```python
from build123d import *

# Parameters (mm, degrees)
BOSS_EXTRU_1_DEPTH                       = 28.5
ESQUISSE5_W                              = 45
ESQUISSE5_H                              = 12.6
BOSS_EXTRU_2_DEPTH                       = 9
ESQUISSE3_R                              = 24.1
ENL_V_MAT_EXTRU_3_DEPTH                  = 8
ENL_V_START                              = -12.6
ENL_V_MAT_EXTRU_5_DEPTH                  = 12.6
ENL_V_START_2                            = -1
ESQUISSE4_R                              = 24.1
ESQUISSE4_R_2                            = 8.05
ENL_V_MAT_EXTRU_4_DEPTH                  = 1
ENL_V_MAT_EXTRU_7_DEPTH                  = 161.796665884
ENL_V_MAT_EXTRU_7_DEPTH_BACK             = 161.796665884
ENL_V_START_3                            = -4
ESQUISSE8_R                              = 7.5
ENL_V_MAT_EXTRU_8_DEPTH                  = 26
ENL_V_START_4                            = 8
ESQUISSE9_R                              = 15
ENL_V_MAT_EXTRU_9_DEPTH                  = 10
ESQUISSE10_R                             = 15
ESQUISSE10_R_2                           = 8.05
ENL_V_MAT_EXTRU_10_DEPTH                 = 1
CONG_1_R                                 = 2
ESQUISSE11_W                             = 12
ESQUISSE11_H                             = 8
ENL_V_MAT_EXTRU_11_DEPTH                 = 23.5
CONG_2_R                                 = 1
FRAISAGE_POUR_VIS_T_TE_FRAIS_E_6_2_COUNT = 2
FRAISAGE_POUR_VIS_T_TE_FRAIS_E_6_2_PITCH = 48
ESQUISSE16_R                             = 1.35
ENL_V_MAT_EXTRU_12_DEPTH                 = 7
BOSS_EXTRU_4_START                       = 1.75
BOSS_EXTRU_4_DEPTH                       = 1.75
BOSS_EXTRU_5_DEPTH                       = 1.75
CHANFREIN2_ANGLE                         = 177.039506
CHANFREIN1_SIZE                          = 1.5


with BuildPart() as part:
    # Esquisse1 → Boss.-Extru.1 (new body)
    with BuildSketch(Plane(origin=(0, -156.353982231, 0), x_dir=(1, 0, 0), z_dir=(0, 1, 0))):
        with BuildLine():
            Line((16.5, -20), (16.5, 20))
            ThreePointArc((16.5, 20), (15.792893219, 20.292893219), (15.5, 21))
            Line((15.5, 21), (15.5, 24))
            ThreePointArc((15.5, 24), (11.5, 28), (7.5, 24))
            Line((7.5, 24), (7.5, 18.75))
            Line((7.5, 18.75), (7.5, 17))
            ThreePointArc((7.5, 17), (7.207106781, 16.292893219), (6.5, 16))
            Line((6.5, 16), (-12, 16))
            ThreePointArc((-12, 16), (-12.707106781, 16.292893219), (-13, 17))
            Line((-13, 17), (-13, 24))
            ThreePointArc((-13, 24), (-17, 28), (-21, 24))
            Line((-21, 24), (-21, 21))
            ThreePointArc((-21, 21), (-21.292893219, 20.292893219), (-22, 20))
            Line((-22, 20), (-25, 20))
            Line((-25, 20), (-25, -20))
            Line((-25, -20), (-22, -20))
            ThreePointArc((-22, -20), (-21.292893219, -20.292893219), (-21, -21))
            Line((-21, -21), (-21, -24))
            ThreePointArc((-21, -24), (-17, -28), (-13, -24))
            Line((-13, -24), (-13, -13))
            ThreePointArc((-13, -13), (-12.707106781, -12.292893219), (-12, -12))
            Line((-12, -12), (6.5, -12))
            ThreePointArc((6.5, -12), (7.207106781, -12.292893219), (7.5, -13))
            Line((7.5, -13), (7.5, -24))
            ThreePointArc((7.5, -24), (11.5, -28), (15.5, -24))
            Line((15.5, -24), (15.5, -21))
            ThreePointArc((15.5, -21), (15.792893219, -20.292893219), (16.5, -20))
        make_face()
    extrude(amount=BOSS_EXTRU_1_DEPTH)

    # Esquisse5 → Boss.-Extru.2 (add)
    with BuildSketch(Plane(origin=(0, -127.853982231, 0), x_dir=(1, 0, 0), z_dir=(0, 1, 0))):
        with Locations((-2.5, 7.3)):
            Rectangle(ESQUISSE5_W, ESQUISSE5_H)
    extrude(amount=BOSS_EXTRU_2_DEPTH)

    # Esquisse3 → Enlèv. mat.-Extru.3 (cut)
    with BuildSketch(Plane(origin=(0, -128.853982231, -11), x_dir=(1, 0, 0), z_dir=(0, 0, 1))):
        with Locations((0, -15.5)):
            Circle(ESQUISSE3_R)
    extrude(amount=ENL_V_MAT_EXTRU_3_DEPTH, mode=Mode.SUBTRACT)

    # Esquisse6 → Enlèv. mat.-Extru.5 (cut)
    with BuildSketch(Plane.XY.offset(-1).offset(ENL_V_START)):
        Polygon((-25, -104.147876216), (-25, -127.853982231), (-21, -127.853982231), (-21, -123.853982231), (-6, -118.853982231), (6, -118.853982231), (20, -123.853982231), (20, -104.147876216), align=None)
    extrude(amount=ENL_V_MAT_EXTRU_5_DEPTH, mode=Mode.SUBTRACT)

    # Esquisse4 → Enlèv. mat.-Extru.4 (cut)
    with BuildSketch(Plane(origin=(0, -168.853982231, -11), x_dir=(1, 0, 0), z_dir=(0, 0, 1)).offset(ENL_V_START_2)):
        with Locations((0, 24.5)):
            Circle(ESQUISSE4_R)
        with Locations((0, 24.5)):
            Circle(ESQUISSE4_R_2, mode=Mode.SUBTRACT)
    extrude(amount=ENL_V_MAT_EXTRU_4_DEPTH, mode=Mode.SUBTRACT)

    # Esquisse7 → Enlèv. mat.-Extru.7 (cut, two sides: drawn at the far end of the back side and taken through both)
    with BuildSketch(Plane.XY.offset(-ENL_V_MAT_EXTRU_7_DEPTH_BACK)):
        with BuildLine():
            Line((-4.030508653, -148.384490884), (-12, -156.353982231))
            Line((-12, -156.353982231), (16.5, -156.353982231))
            Line((16.5, -156.353982231), (16.5, -127.853982231))
            Line((16.5, -127.853982231), (4.030508653, -140.323473578))
            ThreePointArc((4.030508653, -140.323473578), (-4.030508653, -140.323473578), (-4.030508653, -148.384490884))
        make_face()
    extrude(amount=ENL_V_MAT_EXTRU_7_DEPTH + ENL_V_MAT_EXTRU_7_DEPTH_BACK, mode=Mode.SUBTRACT)

    # Esquisse8 → Enlèv. mat.-Extru.8 (cut)
    with BuildSketch(Plane.XY.offset(-11).offset(ENL_V_START_3)):
        with Locations((0, -144.353982231)):
            Circle(ESQUISSE8_R)
    extrude(amount=ENL_V_MAT_EXTRU_8_DEPTH, mode=Mode.SUBTRACT)

    # Esquisse9 → Enlèv. mat.-Extru.9 (cut)
    with BuildSketch(Plane.XY.offset(-11).offset(ENL_V_START_4)):
        with Locations((0, -144.353982231)):
            Circle(ESQUISSE9_R)
    extrude(amount=ENL_V_MAT_EXTRU_9_DEPTH, mode=Mode.SUBTRACT)

    # Esquisse10 → Enlèv. mat.-Extru.10 (cut)
    with BuildSketch(Plane(origin=(0, 0, 7), x_dir=(-1, 0, 0), z_dir=(0, 0, -1)).offset(ENL_V_START_2)):
        with Locations((0, -144.353982231)):
            Circle(ESQUISSE10_R)
        with Locations((0, -144.353982231)):
            Circle(ESQUISSE10_R_2, mode=Mode.SUBTRACT)
    extrude(amount=ENL_V_MAT_EXTRU_10_DEPTH, mode=Mode.SUBTRACT)

    # Congé1
    # the kernel refuses this fillet: 2 mm, written as the material it adds along each edge
    with BuildSketch(Plane(origin=(0, -144.353982231, -12), x_dir=(0.7071067811865527, 0.7071067811865425, 0), z_dir=(0.7071067811865425, -0.7071067811865527, 0))) as cong_1_piece_1:
        with BuildLine():
            CenterArc((9.782050808, 2), CONG_1_R, 210, 60)
            Line((9.782050808, 0), (8.05, 0))
            Line((8.05, 0), (8.05, 1))
        make_face()
    revolve(axis=Axis((0, -144.353982231, -12), (0, 0, 1)), revolution_arc=180)
    with BuildSketch(Plane(origin=(0, -144.353982231, 8), x_dir=(0.7071067811865495, 0.7071067811865456, 0), z_dir=(0.7071067811865456, -0.7071067811865495, 0))) as cong_1_piece_2:
        with BuildLine():
            CenterArc((9.782050808, -2), CONG_1_R, 90, 60)
            Line((8.05, -1), (8.05, 0))
            Line((8.05, 0), (9.782050808, 0))
        make_face()
    revolve(axis=Axis((0, -144.353982231, 8), (0, 0, 1)), revolution_arc=180)
    # the kernel refuses this fillet: 2 mm, written as the material it takes off along each edge
    with BuildSketch(Plane(origin=(0, -144.353982231, -3), x_dir=(0.8997810894111481, 0.43634159913774845, 0), z_dir=(0.43634159913774845, -0.8997810894111481, 0))) as cong_1_2_piece_1:
        with BuildLine():
            CenterArc((15 + CONG_1_R, CONG_1_R), CONG_1_R, 180, 90)
            Line((15 + CONG_1_R, 0), (15, 0))
            Line((15, 0), (15, CONG_1_R))
        make_face()
    revolve(axis=Axis((0, -144.353982231, -3), (0, 0, 1)), revolution_arc=218.25861464, mode=Mode.SUBTRACT)

    # Esquisse11 → Enlèv. mat.-Extru.11 (cut)
    with BuildSketch(Plane(origin=(0, -127.853982231, 0), x_dir=(1, 0, 0), z_dir=(0, 1, 0))):
        with Locations((-19, 24)):
            Rectangle(ESQUISSE11_W, ESQUISSE11_H)
        with Locations((-19, -24)):
            Rectangle(ESQUISSE11_W, ESQUISSE11_H)
    extrude(amount=-ENL_V_MAT_EXTRU_11_DEPTH, mode=Mode.SUBTRACT)

    # Congé2
    cong_2_edges = [part.edges().sort_by_distance(p)[0] for p in [
        (-17.5, -151.353982231, -20),
        (-17.5, -151.353982231, 20),
    ]]
    fillet(cong_2_edges, radius=CONG_2_R)

    # Esquisse12 → Fraisage pour vis _ t_te frais_e _ 6 pan (revolve, cut)
    with BuildSketch(Plane(origin=(-17, -151.353982231, -24), x_dir=(0, 0, 1), z_dir=(1, 0, 0))):
        Polygon((0, 0), (0, 5), (1.6, 5), (1.6, 1.7), (2.9, 0.4), (2.9, 0), align=None)
    fraisage_pour_vis_t_te_frais_e_6_pan = revolve(axis=Axis((-17, -145.003982231, -24), (0, -1, 0)), mode=Mode.SUBTRACT)

    # Fraisage pour vis _ t_te frais_e _ 6 2: Fraisage pour vis _ t_te frais_e _ 6 pan ×2
    with Locations(*[(0, 0, i * FRAISAGE_POUR_VIS_T_TE_FRAIS_E_6_2_PITCH) for i in range(1, FRAISAGE_POUR_VIS_T_TE_FRAIS_E_6_2_COUNT)]):
        add(fraisage_pour_vis_t_te_frais_e_6_pan, mode=Mode.SUBTRACT)

    # Fraisage pour vis _ t_te frais_e _ 6 3: read off the stored shape, not the designer's step
    # Fraisage pour vis _ t_te frais_e _ 6 3 o → Fraisage pour vis _ t_te frais_e _ 6 3 (revolve, cut)
    with BuildSketch(Plane(origin=(11.5, 0, 24), x_dir=(1, 0, 0), z_dir=(0, 0, 1))):
        Polygon((0, -134.475881673), (1.6, -134.475881673), (1.6, -129.553982231), (2.9, -128.253982231), (2.9, -127.853982231), (0, -127.853982231), align=None)
    revolve(axis=Axis((11.5, 0, 24), (0, 1, 0)), mode=Mode.SUBTRACT)

    # Fraisage pour vis _ t_te frais_e _ 6 4 → Fraisage pour vis _ t_te frais_e _ 6 3 2 (revolve, cut)
    with BuildSketch(Plane(origin=(11.5, 0, -24), x_dir=(1, 0, 0), z_dir=(0, 0, 1))):
        Polygon((0, -134.475881673), (1.6, -134.475881673), (1.6, -129.553982231), (2.9, -128.253982231), (2.9, -127.853982231), (0, -127.853982231), align=None)
    revolve(axis=Axis((11.5, 0, -24), (0, 1, 0)), mode=Mode.SUBTRACT)

    # Esquisse16 → Enlèv. mat.-Extru.12 (cut)
    with BuildSketch(Plane(origin=(0, -127.853982231, 0), x_dir=(1, 0, 0), z_dir=(0, 1, 0))):
        with Locations(Location((-21, 16.8, 0), (0, 0, 180))):
            Circle(ESQUISSE16_R)
        with Locations(Location((11.5, 16.8, 0), (0, 0, 180))):
            Circle(ESQUISSE16_R)
        with Locations((11.5, -16.8)):
            Circle(ESQUISSE16_R)
        with Locations((-21, -16.8)):
            Circle(ESQUISSE16_R)
    extrude(amount=-ENL_V_MAT_EXTRU_12_DEPTH, mode=Mode.SUBTRACT)

    # Esquisse17 → Boss.-Extru.4 (add)
    with BuildSketch(Plane(origin=(0, 0, -16), x_dir=(-1, 0, 0), z_dir=(0, 0, -1)).offset(BOSS_EXTRU_4_START)):
        with BuildLine():
            Line((-4.030508653, -140.323473578), (-7.919595949, -136.434386282))
            ThreePointArc((-7.919595949, -136.434386282), (7.919595949, -136.434386282), (7.919595949, -152.27357818))
            Line((7.919595949, -152.27357818), (4.030508653, -148.384490884))
            ThreePointArc((4.030508653, -148.384490884), (4.030508653, -140.323473578), (-4.030508653, -140.323473578))
        make_face()
    extrude(amount=-BOSS_EXTRU_4_DEPTH)

    # Esquisse18 → Boss.-Extru.5 (add)
    with BuildSketch(Plane.XY.offset(12)):
        with BuildLine():
            Line((7.919595949, -136.434386282), (4.030508653, -140.323473578))
            ThreePointArc((4.030508653, -140.323473578), (-4.030508653, -140.323473578), (-4.030508653, -148.384490884))
            Line((-4.030508653, -148.384490884), (-7.919595949, -152.27357818))
            ThreePointArc((-7.919595949, -152.27357818), (-7.919595949, -136.434386282), (7.919595949, -136.434386282))
        make_face()
    extrude(amount=BOSS_EXTRU_5_DEPTH)

    # Chanfrein2: read off the stored shape, not the designer's step
    # Chanfrein2 outline → Chanfrein2 (revolve)
    with BuildSketch(Plane(origin=(0, -144.353982231, 0), x_dir=(0.66964285714286, 0.742683272921605, 0), z_dir=(0.742683272921605, -0.66964285714286, 0))):
        Polygon((13.7, 12), (11.2, 13.75), (11.2, 12), align=None)
        Polygon((11.2, -17.75), (13.7, -16), (11.2, -16), align=None)
    revolve(axis=Axis((0, -144.353982231, 0), (0, 0, 1)), revolution_arc=CHANFREIN2_ANGLE)

    # Chanfrein1
    chanfrein1_edges = [part.edges().sort_by_distance(p)[0] for p in [
        (-4.030508653, -140.323473578, -17.75),
        (-4.030508653, -140.323473578, 13.75),
    ]]
    chamfer(chanfrein1_edges, length=CHANFREIN1_SIZE)


solid = part.part
```
Here's how the part is built. I have some questions about the finished solid (model axes, mm). A direction names the side the tool comes from. Coordinates: 2 decimals unless noted, no trailing zeros. Write each loop counter-clockwise with the first axis right and the second up, starting at its lowest first coordinate (ties: lowest second). Pieces come first, ordered by that corner, then holes. Notation, with made-up numbers: (-33, 37.25) - (-1, 37.25) arc R27 ccw to (-1, 69.25) - close; hole circle Ø7 at (14, 60.5). An arc over 180 degrees is marked (long way). One line per item, written item: value.
1) Suppose I cut it at B-B on z = 0.5. Write out the boundary of the cut face in (x, y).
Model answer:
outline: (-25, -156.35) - (-12, -156.35) - (-10.61, -154.96) arc R15 cw to (10.61, -133.75) - (16.5, -127.85) - (-25, -127.85) - close
2) We'd pull the mould along Y, two halves only. Please class faces 4 (the cylindrical face through (-5.19, -138.94, -13.03)), 5 (the flat face through (11.738, -132.616, 12.717)), 6 (the cylindrical face through (-15.235, -151.551, -26.301)), 7 (the cylindrical face through (-3.941, -140.236, 11.616)): pulls with the +Y half, pulls with the -Y half, needs draft (parallel to the pull), parting line crosses it, or undercut.
Model answer:
face 4: undercut
face 5: pulls with the -Y half
face 6: needs draft
face 7: undercut
3) I'm going to push flat-ended pins straight in: P1, Ø2.5, axis at x = 11.5, z = -16.8, coming from the -Y side; P2, Ø2, axis at y = -148.5, z = -19.5, coming from the +X side; P3, Ø1.5, axis at x = -5.5, z = -14, coming from the -Y side; P4, Ø12, axis at x = 14.5, z = 1.5, coming from the +Y side. Where does each tip first touch, or does it pass through?
Model answer:
P1: passes through
P2: stops at x = -13
P3: stops at y = -150.6
P4: stops at y = -119.94
4) I need wall thicknesses on line 1 along X through (y, z) = (-133.5, 16.8); line 2 along Z through (x, y) = (-21, -130); line 3 along Z through (x, y) = (2, -124). Which ranges of each line are inside material? Lowest first, please.
Model answer:
line 1: x = -25 to -22.35, -19.65 to -13, 7.5 to 10.15
line 2: z = -20 to -18.15, -15.45 to 15.45, 18.15 to 20
line 3: z = -13.6 to -12, -3 to -1
5) On a 3-axis mill with a long thin cutter (end or side, diameter ignored), from which of +Z, -Z, +X, -X, +Y, -Y can I reach the whole of each face in a straight line? I mean faces 1 (the flat face through (-18, -151.354, 27)), 2 (the flat face through (-5, -138, 13.75)), 3 (the flat face through (-19, -139, 20)). Say none if no direction works.
Model answer:
face 1: +Z, +X, -X, +Y
face 2: +Z, +Y, -Y
face 3: +Z, -X, +Y
